Could you check a few things on this drawing? It's one solid part, dimensions in mm from its lowest x, y, z. A direction names the side the tool comes from. Give positions to 0.01 mm unless a question says otherwise; leave off trailing zeros. Loops run counter-clockwise (first coordinate to the right, second up) from the corner with the lowest first, then second, coordinate; pieces in that order, holes last. Notation, with made-up numbers: M 48.5,59.25 L 56.5,59.25 A30 cw 56.5,87.25 Z; hole C -19.75,31.5 d10. An arc over 180 degrees is marked long. Answer as CSV lines item,"result". Start each with the question number.
Item 1: I want a section at A-A on z = 75. List the corners of the cut face in (x, y) for me.
Item 2: Will these pins go through, and if not, where does the flat tip stop? P1, Ø6.5, axis at x = 40, z = 75, coming from the -Y side; P2, Ø1.5, axis at y = 2, z = 9.5, coming from the -X side.
Item 3: I want a section at C-C on y = 5. Give the number of separate pieces and of enclosed holes in the cut face, plus the area to 3 significant figures.
Item 4: If I drill on line 1 along X through (y, z) = (0.6, 40); line 2 along X through (y, z) = (4.5, 40); line 3 along X through (y, z) = (8.5, 15.5) (1 decimal), over which ranges is the centre line in solid material (lowest first)? Write a range as from..to.
Item 5: I want a section at D-D on z = 15. List the corners of the cut face in (x, y) for me (1 decimal), plus the area to 3 significant figures.
Item 6: I want a section at B-B on x = 40. List the corners of the cut face in (y, z) for me, plus the area to 3 significant figures.
Item 7: For the marked faces 1 and 2, which set-ups out of +Z, -Z, +X, -X, +Y, -Y let a thin tool reach every point of the face, with its end or its side?
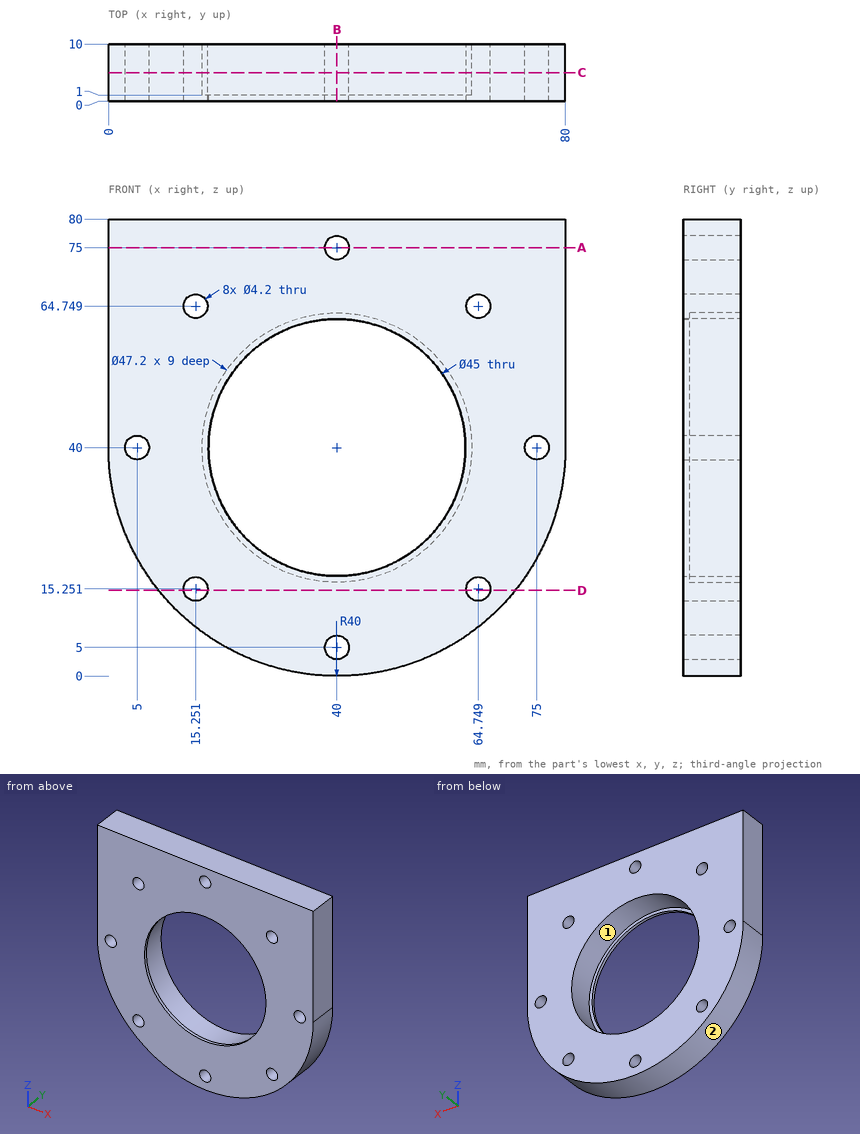
Result:
1,outline,"M 0,0 L 37.9,0 L 37.9,10 L 0,10 Z; M 42.1,0 L 80,0 L 80,10 L 42.1,10 Z"
2,P1,"y = 0"
2,P2,"x = 13.26"
3,separate pieces,"1"
3,enclosed holes,"9"
3,area,"3,850 mm^2"
4,line 1,"0..2.9, 7.1..17.5, 62.5..72.9, 77.1..80"
4,line 2,"0..2.9, 7.1..16.4, 63.6..72.9, 77.1..80"
4,line 3,"8.4..13.2, 17.3..62.7, 66.8..71.6"
5,outline,"M 8.8,0 L 13.2,0 L 13.2,10 L 8.8,10 Z; M 17.3,0 L 62.7,0 L 62.7,10 L 17.3,10 Z; M 66.8,0 L 71.2,0 L 71.2,10 L 66.8,10 Z"
5,area,"541 mm^2"
6,outline,"M 0,0 L 10,0 L 10,2.9 L 0,2.9 Z; M 0,7.1 L 10,7.1 L 10,16.4 L 1,16.4 L 1,17.5 L 0,17.5 Z; M 0,62.5 L 1,62.5 L 1,63.6 L 10,63.6 L 10,72.9 L 0,72.9 Z; M 0,77.1 L 10,77.1 L 10,80 L 0,80 Z"
6,area,"246 mm^2"
7,face 1,"+Y"
7,face 2,"-Z, +Y, -Y"
